Autodesk Inventor part; units mm, degrees
ref_plane "YZ Plane" through (0, 0, 0) normal (1, 0, 0) x (0, 1, 0)
ref_plane "XZ Plane" through (0, 0, 0) normal (0, 1, 0) x (-1, 0, 0)
ref_plane "XY Plane" through (0, 0, 0) normal (0, 0, 1) x (1, 0, 0)
sketch "Sketch1" plane through (0, 0, 0) normal (0, 0, 1) x (1, 0, 0)
  circle A0 centre (0, 0) radius 8.5
  dimension "d0" = 17
extrude "Extrusion1" add sketch "Sketch1" against normal blind 51.2
sketch "Sketch2" plane through (0, 0, 0) normal (0, 0, 1) x (1, 0, 0)
  circle A0 centre (0, 0) radius 6.75
  dimension "d3" = 13.5
extrude "Extrusion2" add sketch "Sketch2" along normal blind 25.3
sketch "Sketch3" plane through (0, 0, -51.2) normal (0, 0, -1) x (-1, 0, 0)
  circle A0 centre (0, 0) radius 9.5
  dimension "d6" = 19
extrude "Extrusion3" add sketch "Sketch3" along normal blind 20.4952
sketch "Sketch4" plane through (0, 0, -71.6952) normal (0, 0, -1) x (-1, 0, 0)
  circle A0 centre (0, 0) radius 17.15
  dimension "d9" = 34.3
extrude "Extrusion4" add sketch "Sketch4" along normal blind 5
properties part number "spindle"
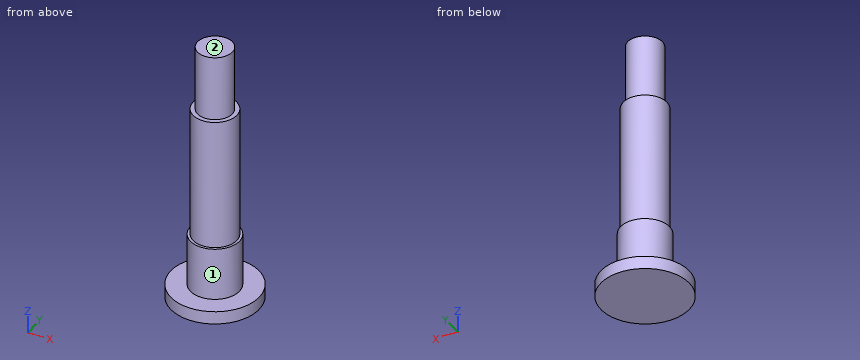
Part model, mm, in its own coordinate system. Face numbers are marked on the shaded views. A direction names the side the tool comes from. Coordinates: 2 decimals unless noted, no trailing zeros. Order: outer loops, then holes, each group sorted by start corner. A loop starts at its lowest first (then second) coordinate and runs counter-clockwise, first axis right, second up. Notation, with made-up numbers: (-36.5, 54.5) - (4.5, 54.5) arc R31 cw to (4.5, 87.5) - close; hole circle Ø8 at (75.25, -7.5). An arc over 180 degrees is marked (long way). Return JSON: item names as keys, results as strings. Group by question number.
Item 1: Cut at D-D (x = -12.5). List the corners of the cut face in (y, z).
Item 2: Cut at C-C (z = -53). List the corners of the cut face in (x, y).
Item 3: Pin check, flat tips, straight feed: pin 1 (6 mm diameter, centred on x = 10.5, z = -53, fed in from -Y); pin 2 (10 mm diameter, centred on y = 1.5, z = -42.5, fed in from -X); pin 3 (5 mm diameter, centred on x = 9.5, z = -41, fed in from +Y). Stop position of each tip, or through.
Item 4: Which spindle directions (+Z, -Z, +X, -X, +Y, -Y) get a long thin tool onto all of the face, cutting with end or side? Do the marked faces 1 and 2. Say none if no direction does.
Item 5: Cut at A-A (x = 0). List the corners of the cut face in (y, z).
Item 6: Drill centre lines: probe 1 along Z at (x, y) = (15, -1); probe 2 along X at (y, z) = (-0.5, -62.5); probe 3 along Z at (x, y) = (-5, 5). Where is each one in solid material? Low to high. Write a range as from..to.
Check values:
{
 "1": {"outline": "(-11.74, -76.7) - (11.74, -76.7) - (11.74, -71.7) - (-11.74, -71.7) - close"},
 "2": {"outline": "circle Ø19 at (0, 0)"},
 "3": {"pin 1": "stops at y = -5.83", "pin 2": "stops at x = -8.5", "pin 3": "stops at y = 4.82"},
 "4": {"face 1": "+Z", "face 2": "+Z, +X, -X, +Y, -Y"},
 "5": {"outline": "(-17.15, -76.7) - (17.15, -76.7) - (17.15, -71.7) - (9.5, -71.7) - (9.5, -51.2) - (8.5, -51.2) - (8.5, 0) - (6.75, 0) - (6.75, 25.3) - (-6.75, 25.3) - (-6.75, 0) - (-8.5, 0) - (-8.5, -51.2) - (-9.5, -51.2) - (-9.5, -71.7) - (-17.15, -71.7) - close"},
 "6": {"probe 1": "z = -76.7..-71.7", "probe 2": "x = -9.49..9.49", "probe 3": "z = -76.7..0"}
}
